Read the model definition and answer for the solid it produces. Units are mm, in the model's axes. Coordinates: 2 decimals unless noted, no trailing zeros. Order: outer loops, then holes, each group sorted by start corner. A loop starts at its lowest first (then second) coordinate and runs counter-clockwise, first axis right, second up. Notation, with made-up numbers: M 83,6.25 L 122,6.25 A21 ccw 122,23.25 Z; hole C 5.5,-29 d6. An arc over 180 degrees is marked long. Use a Markdown table: item, result. Add a question column.
1) Each of these flat-tipped pins is pushed along its axis until it touches: pin 1 Ø2 at (x, z) = (-24.5, 9) entering from -Y; pin 2 Ø3 at (x, z) = (-8, 6.5) entering from +Y; pin 3 Ø3 at (x, y) = (0, -14) entering from +Z; pin 4 Ø1 at (y, z) = (-14, 11.5) entering from -X. Where does it stop, or does it pass through?
2) Find the intervals of material crossed by probe 1 along Y at (x, z) = (0, 9); probe 2 along Y at (x, z) = (14, 9); probe 3 along Y at (x, z) = (2.5, 15), in increasing order. Write a range as [from, to].
3) Find section C-C on x = 14. Write down the section's boundary in (y, z).
4) Find section D-D on z = 5.5. Write down the section's boundary in (x, y), plus the area to 3 significant figures.
5) Find section A-A on y = 0. Write down the section's boundary in (x, z), plus the area to 3 significant figures.
6) The mould has two halves that part along X. Classify faces 1 (the face through (8, 1, 20)), 2 (the face through (-1.216, 15.115, 9.86)), 3 (the face through (-8.67, -39.05, 9.86)), 4 (the face through (15.524, -0.632, 9.86)): released by +X, released by -X, zero draft, split by the parting line, or undercut.
from build123d import *

# Parameters (mm, degrees)
F0_R     = 40
F0_R_2   = 7.5
F2_DEPTH = 20
F1_R     = 1.65
F3_DEPTH = 20


with BuildPart() as f2:
    # F0 (on Top) → F2 (new body)
    with BuildSketch(Plane.XY):
        Circle(F0_R)
        Circle(F0_R_2, mode=Mode.SUBTRACT)
    extrude(amount=F2_DEPTH)

    # F1 (on Top) → F3 (cut)
    with BuildSketch(Plane.XY):
        with Locations((0, -14)):
            Circle(F1_R)
        with Locations((14, 0)):
            Circle(F1_R)
        with Locations((0, 14)):
            Circle(F1_R)
        with Locations((-14, 0)):
            Circle(F1_R)
    extrude(amount=F3_DEPTH, mode=Mode.SUBTRACT)


solid = f2.part
Check result:
| question | item | result |
|---|---|---|
| 1 | pin 1 | stops at y = -32.37 |
| 1 | pin 2 | stops at y = 39.47 |
| 1 | pin 3 | passes through |
| 1 | pin 4 | stops at x = -37.65 |
| 2 | probe 1 | y = [-40, -15.65], [-12.35, -7.5], [7.5, 12.35], [15.65, 40] |
| 2 | probe 2 | y = [-37.47, -1.65], [1.65, 37.47] |
| 2 | probe 3 | y = [-39.92, -7.07], [7.07, 39.92] |
| 3 | outline | M -37.47,0 L -1.65,0 L -1.65,20 L -37.47,20 Z; M 1.65,0 L 37.47,0 L 37.47,20 L 1.65,20 Z |
| 4 | outline | C 0,0 d80; hole C -14,0 d3.3; hole C 0,0 d15; hole C 0,-14 d3.3; hole C 0,14 d3.3; hole C 14,0 d3.3 |
| 4 | area | 4,820 mm2 |
| 5 | outline | M -40,0 L -15.65,0 L -15.65,20 L -40,20 Z; M -12.35,0 L -7.5,0 L -7.5,20 L -12.35,20 Z; M 7.5,0 L 12.35,0 L 12.35,20 L 7.5,20 Z; M 15.65,0 L 40,0 L 40,20 L 15.65,20 Z |
| 5 | area | 1,170 mm2 |
| 6 | face 1 | zero draft |
| 6 | face 2 | undercut |
| 6 | face 3 | split by the parting line |
| 6 | face 4 | undercut |
